For this review, take the finished solid that the model builds, in its own axes (mm). A direction names the side the tool comes from. Coordinates: 2 decimals unless noted, no trailing zeros. Loops run counter-clockwise (first coordinate to the right, second up) from the corner with the lowest first, then second, coordinate; pieces in that order, holes last. Notation, with made-up numbers: M 21.5,13 L 78.5,13 A32 cw 78.5,51 Z; hole C 46,33 d10. An arc over 180 degrees is marked long. Answer as a JSON object with one key per item and string values. Group by question number.
Item 1: Mouldability with a two-part tool opening along X and no side actions: class faces 5 (the face through (-10, -8, 7)), 6 (the face through (-23, 1, 17)), 7 (the face through (-24.7, -10.5, 5.1)) as +X half, -X half, draft (parallel to the pull), parting line (faces both ways), or undercut.
Item 2: Tool access review of faces 1 (the face through (-26, -34, -2)), 2 (the face through (-23, 1, -8)), 3 (the face through (-28, -34, 0)), 4 (the face through (-28, -31, -5)): name each direction out of +Z, -Z, +X, -X, +Y, -Y from which nothing blocks a thin tool from reaching the whole face with its end or side.
Item 3: Add section B-B (y = -48.24). State the section outline as (x, z) points, then the cut area to 3 significant figures.
Item 4: Add section A-A (x = 27.5). State the section outline as (y, z) points.
Item 5: Insertion check: pin 1 (2.5 mm diameter, centred on y = 1.5, z = 18, fed in from -X); pin 2 (8 mm diameter, centred on y = -37.5, z = -6.5, fed in from -X); pin 3 (10 mm diameter, centred on x = 9.5, y = -16, fed in from +Z); pin 4 (8.5 mm diameter, centred on x = -7.5, z = 5, fed in from -Y). Each pin has a flat end and moves straight along its axis. Give the tip position at first contact, or say it passes through.
Item 6: Add section C-C (x = -27.5). Count the separate pieces of the cut face and the enclosed holes in it, then the cut area to 3 significant figures.
Item 7: Wall thickness on L1, parallel to X at y = 2.3, z = -9.4; L2, parallel to X at y = 2.1, z = 9.4; L3, parallel to X at y = -7.5, z = -15: over which ranges is each line inside the solid? List them lowest first. Write a range as from..to.
Item 8: Add section D-D (z = 9.4). State the section outline as (x, y) points, then the cut area to 3 significant figures.
from build123d import *

# Parameters (mm, degrees)
SKETCH_1_W          = 9
SKETCH_1_H          = 40
SKETCH_1_R          = 1.7
EXTRUDE_1_DEPTH     = 3
EXTRUDE_1_2_DEPTH   = 3
SKETCH_2_W          = 46
SKETCH_2_H          = 10
EXTRUDE_2_DEPTH     = 3
SKETCH_3_W          = 22
SKETCH_3_H          = 10
EXTRUDE_3_DEPTH     = 8
EXTRUDE_5_DEPTH     = 5
SKETCH_11_W         = 30
SKETCH_11_H         = 52
EXTRUDE_6_DEPTH     = 3
SKETCH_12_R         = 2.1
SKETCH_12_R_2       = 2.25
CUT_EXTRUDE_3_DEPTH = 13
SKETCH_13_W         = 25
SKETCH_13_H         = 28.4
CUT_EXTRUDE_4_DEPTH = 13
CHAMFER_3_SIZE      = 10
CHAMFER_4_SIZE      = 5
CHAMFER_5_SIZE      = 5
SKETCH_14_W         = 22.803508502
SKETCH_14_H         = 5
EXTRUDE_7_DEPTH     = 5
EXTRUDE_8_REACH     = 78.026
SKETCH_15_W         = 3.946761087
SKETCH_15_H         = 5
CHAMFER_6_SIZE      = 5
EXTRUDE_9_DEPTH     = 5


with BuildPart() as part:
    # Sketch 1 → Extrude 1 (new body)
    with BuildSketch(Plane(origin=(0, 0, 0), x_dir=(1, 0, 0), z_dir=(0, 1, 0))):
        with Locations((27.5, 0)):
            Rectangle(SKETCH_1_W, SKETCH_1_H)
        with Locations(Location((27.5, 9.4, 0), (0, 0, 90))):
            Circle(SKETCH_1_R, mode=Mode.SUBTRACT)
        with Locations(Location((27.5, -9.4, 0), (0, 0, 270))):
            Circle(SKETCH_1_R, mode=Mode.SUBTRACT)
    extrude(amount=EXTRUDE_1_DEPTH)



with BuildPart() as body_2:
    # Sketch 1 → Extrude 1 2 (new body)
    with BuildSketch(Plane(origin=(0, 0, 0), x_dir=(1, 0, 0), z_dir=(0, 1, 0))):
        with Locations((-27.5, 0)):
            Rectangle(SKETCH_1_W, SKETCH_1_H)
        with Locations(Location((-27.5, 9.4, 0), (0, 0, 270))):
            Circle(SKETCH_1_R, mode=Mode.SUBTRACT)
        with Locations(Location((-27.5, -9.4, 0), (0, 0, 90))):
            Circle(SKETCH_1_R, mode=Mode.SUBTRACT)
    extrude(amount=EXTRUDE_1_2_DEPTH)


with BuildPart() as part_1:
    add(part.part)

    add(body_2.part)  # Extrude 2 merges body 2
    # Sketch 2 → Extrude 2 (add)
    with BuildSketch(Plane(origin=(0, 0, 0), x_dir=(-1, 0, 0), z_dir=(0, -1, 0))):
        with Locations((0, -9)):
            Rectangle(SKETCH_2_W, SKETCH_2_H)
    extrude(amount=-EXTRUDE_2_DEPTH)

    # Sketch 3 → Extrude 3 (add)
    with BuildSketch(Plane.XZ):
        with Locations((0, 9)):
            Rectangle(SKETCH_3_W, SKETCH_3_H)
    extrude(amount=EXTRUDE_3_DEPTH)

    # Sketch 10 → Extrude 5 (add)
    with BuildSketch(Plane.XZ.offset(8)):
        Polygon((-11, 14), (-29, 0), (-29, -12.266402166), (-11, 4), align=None)
    extrude(amount=-EXTRUDE_5_DEPTH)

    # Sketch 11 → Extrude 6 (add)
    with BuildSketch(Plane.ZY.offset(29)):
        with Locations((-15, -29)):
            Rectangle(SKETCH_11_W, SKETCH_11_H)
    extrude(amount=-EXTRUDE_6_DEPTH)

    # Sketch 12 → Cut-Extrude 3 (cut)
    with BuildSketch(Plane(origin=(-26, 0, 0), x_dir=(0, 0, -1), z_dir=(1, 0, 0))):
        with Locations((20.414, -13.24)):
            Circle(SKETCH_12_R)
        with Locations((20.414, -48.24)):
            Circle(SKETCH_12_R_2)
    extrude(amount=-CUT_EXTRUDE_3_DEPTH, mode=Mode.SUBTRACT)

    # Sketch 13 → Cut-Extrude 4 (cut)
    with BuildSketch(Plane.ZY.offset(29)):
        with Locations((-17.5, -30.74)):
            Rectangle(SKETCH_13_W, SKETCH_13_H)
    extrude(amount=-CUT_EXTRUDE_4_DEPTH, mode=Mode.SUBTRACT)

    # Chamfer 3
    chamfer_3_edges = [part_1.edges().sort_by_distance(p)[0] for p in [
        (-27.5, -3, -30),
    ]]
    chamfer(chamfer_3_edges, length=CHAMFER_3_SIZE)

    # Chamfer 4
    chamfer_4_edges = [part_1.edges().sort_by_distance(p)[0] for p in [
        (-27.5, -55, -30),
    ]]
    chamfer(chamfer_4_edges, length=CHAMFER_4_SIZE)

    # Chamfer 5
    chamfer_5_edges = [part_1.edges().sort_by_distance(p)[0] for p in [
        (-27.5, -16.54, -5),
        (-27.5, -44.94, -5),
    ]]
    chamfer(chamfer_5_edges, length=CHAMFER_5_SIZE)

    # Sketch 14 → Extrude 7 (add)
    with BuildSketch(Plane(origin=(-10.930769231, 0, 14.053846154), x_dir=(0.7893522173763264, 0, 0.6139406135149205), z_dir=(-0.6139406135149205, 0, 0.7893522173763264))):
        with Locations((-11.489460053, -5.5)):
            Rectangle(SKETCH_14_W, SKETCH_14_H)
    extrude(amount=EXTRUDE_7_DEPTH)

    # Extrude 8: up to this plane
    extrude_8_end = Plane(origin=(-14.000472298, 0, 18.000607241), z_dir=(-0.6139406135149204, 0, 0.7893522173763263))
    # Sketch 15 → Extrude 8 (add, up to the surface)
    with BuildSketch(Plane(origin=(11, 0, 0), x_dir=(0, 0, -1), z_dir=(1, 0, 0)), mode=Mode.PRIVATE) as extrude_8_sk1:
        with Locations((-15.973380544, -5.5)):
            Rectangle(SKETCH_15_W, SKETCH_15_H)
    extrude_8_tool1 = split(extrude(extrude_8_sk1.sketch, amount=-EXTRUDE_8_REACH, mode=Mode.PRIVATE), bisect_by=extrude_8_end, keep=Keep.BOTH, mode=Mode.PRIVATE)
    add(extrude_8_tool1.solids().sort_by_distance((11, -5.5, 15.973381))[0])

    # Chamfer 6
    chamfer_6_edges = [part_1.edges().sort_by_distance(p)[0] for p in [
        (-29, -5.5, 0),
    ]]
    chamfer(chamfer_6_edges, length=CHAMFER_6_SIZE - 0.0001)  # a hair under: the kernel refuses the full size

    # Sketch 17 → Extrude 9 (add)
    with BuildSketch(Plane.XZ.offset(8)):
        Polygon((-29, 0), (-20.325921578, 10.286880116), (-17.338272835, 7.767642096), (-26, -4.155710702), align=None)
    extrude(amount=EXTRUDE_9_DEPTH)


solid = part_1.part
From the geometry:
{
 "1": {"face 5": "draft", "face 6": "undercut", "face 7": "-X half"},
 "2": {"face 1": "-Z, +X, -Y", "face 2": "-Z, +Y", "face 3": "+Z, +X, -X, -Y", "face 4": "-Z, +X, -X"},
 "3": {"outline": "M -29,-30 L -26,-30 L -26,-22.66 L -29,-22.66 Z; M -29,-18.16 L -26,-18.16 L -26,0 L -29,0 Z", "area": "76.5 mm²"},
 "4": {"outline": "M 0,-20 L 3,-20 L 3,-11.1 L 0,-11.1 Z; M 0,-7.7 L 3,-7.7 L 3,7.7 L 0,7.7 Z; M 0,11.1 L 3,11.1 L 3,20 L 0,20 Z"},
 "5": {"pin 1": "stops at x = -32", "pin 2": "stops at x = -29", "pin 3": "passes through", "pin 4": "stops at y = -8"},
 "6": {"separate pieces": "4", "enclosed holes": "2", "area": "929 mm²"},
 "7": {"L1": "x = -32..-29.2, -25.8..-23, 23..25.8, 29.2..32", "L2": "x = -32..-29.2, -25.8..25.8, 29.2..32", "L3": "x = -29..-26"},
 "8": {"outline": "M -32,0 L -29.2,0 L -29.2,3 L -32,3 Z; M -25.8,0 L -11,0 L -11,-3 L -25.06,-3 L -25.06,-8 L -21.07,-8 L -21.07,-13 L -19.27,-13 L -19.27,-8 L 11,-8 L 11,0 L 25.8,0 L 25.8,3 L -25.8,3 Z; M 29.2,0 L 32,0 L 32,3 L 29.2,3 Z", "area": "427 mm²"}
}
